Can you work these out from the model? Positions are in its coordinate system, mm. Give positions to 0.01 mm unless a question says otherwise; leave off trailing zeros. Loops run counter-clockwise (first coordinate to the right, second up) from the corner with the lowest first, then second, coordinate; pieces in that order, holes last. Notation, with made-up numbers: (24.25, -34.5) - (31.25, -34.5) arc R32 ccw to (31.25, -3.5) - close; hole circle Ø1 at (2, 52). An arc over 180 degrees is marked (long way). Use a Markdown table: item, result. Add a question column.
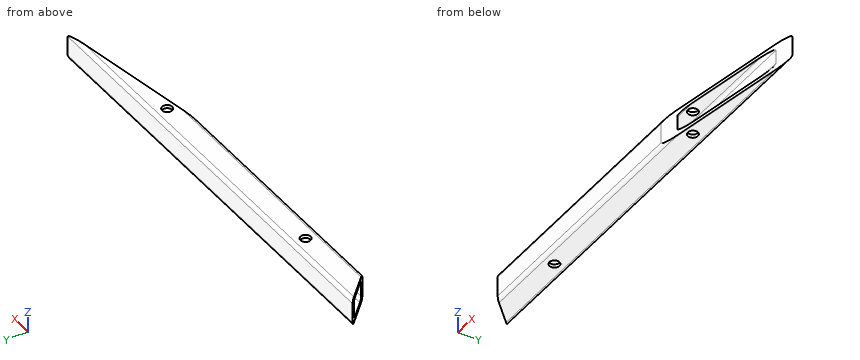
```python
from build123d import *

# Parameters (mm, degrees)
BOSS_EXTRUDE1_DEPTH = 418.338
SKETCH2_R           = 4.7625
CUT_EXTRUDE1_DEPTH  = 420.87736572


with BuildPart() as part:
    # Sketch1 → Boss-Extrude1 (new body)
    with BuildSketch(Plane(origin=(0, 0, 0), x_dir=(0, 0, -1), z_dir=(1, 0, 0))):
        with BuildLine():
            Line((3.302, 0), (22.098, 0))
            ThreePointArc((22.098, 0), (24.432866591, 0.967133409), (25.4, 3.302))
            Line((25.4, 3.302), (25.4, 22.098))
            ThreePointArc((25.4, 22.098), (24.432866591, 24.432866591), (22.098, 25.4))
            Line((22.098, 25.4), (3.302, 25.4))
            ThreePointArc((3.302, 25.4), (0.967133409, 24.432866591), (0, 22.098))
            Line((0, 22.098), (0, 3.302))
            ThreePointArc((0, 3.302), (0.967133409, 0.967133409), (3.302, 0))
        make_face()
        with BuildLine():
            Line((6.223, 3.175), (19.177, 3.175))
            ThreePointArc((19.177, 3.175), (21.332261469, 4.067738531), (22.225, 6.223))
            Line((22.225, 6.223), (22.225, 19.177))
            ThreePointArc((22.225, 19.177), (21.332261469, 21.332261469), (19.177, 22.225))
            Line((19.177, 22.225), (6.223, 22.225))
            ThreePointArc((6.223, 22.225), (4.067738531, 21.332261469), (3.175, 19.177))
            Line((3.175, 19.177), (3.175, 6.223))
            ThreePointArc((3.175, 6.223), (4.067738531, 4.067738531), (6.223, 3.175))
        make_face(mode=Mode.SUBTRACT)
    extrude(amount=BOSS_EXTRUDE1_DEPTH)

    # Sketch2 → Cut-Extrude1 (cut, through all)
    with BuildSketch(Plane.XY):
        with Locations((88.9, 12.7)):
            Circle(SKETCH2_R)
        with Locations((292.1, 12.7)):
            Circle(SKETCH2_R)
        Polygon((0, 0), (0, 25.4), (25.4, 0), align=None)
        Polygon((418.338, 0), (265.303, 0), (418.338, 25.4), align=None)
    extrude(amount=-CUT_EXTRUDE1_DEPTH, mode=Mode.SUBTRACT)


solid = part.part
```
1. Suppose I cut it at B-B (x = 88.9). List the corners of the cut face in (y, z) for me (1 decimal), and give its area (3 significant figures).
2. Please list where these lines run through material, in increasing order: line 1 along Z through (x, y) = (230, 13.5) (3 decimals); line 2 along Y through (x, z) = (88.9, -23.3); line 3 along Y through (x, z) = (292.1, -0.85). Write a range as [from, to].
3. Will these pins go through, and if not, where does the flat tip stop? P1, Ø5, axis at x = 321, z = -7.5, coming from the -Y side; P2, Ø6, axis at x = 352.5, y = 14, coming from the -Z side.
4. Suppose I cut it at A-A (z = -10.25). List the corners of the cut face in (x, y) for me (3 decimals).
5. Suppose I cut it at D-D (x = 292.1). List the corners of the cut face in (y, z) for me (1 decimal), and give its area (3 significant figures).
6. Suppose I cut it at C-C (x = 189). List the corners of the cut face in (y, z) for me (3 decimals), and give its area (3 significant figures).
Results below:
| question | item | result |
|---|---|---|
| 1 | outline | (0, -22.1) arc R3.3 ccw to (3.3, -25.4) - (7.9, -25.4) - (7.9, -22.2) - (6.2, -22.2) arc R3 cw to (3.2, -19.2) - (3.2, -6.2) arc R3 cw to (6.2, -3.2) - (7.9, -3.2) - (7.9, 0) - (3.3, 0) arc R3.3 ccw to (0, -3.3) - close; (17.5, -25.4) - (22.1, -25.4) arc R3.3 ccw to (25.4, -22.1) - (25.4, -3.3) arc R3.3 ccw to (22.1, 0) - (17.5, 0) - (17.5, -3.2) - (19.2, -3.2) arc R3 cw to (22.2, -6.2) - (22.2, -19.2) arc R3 cw to (19.2, -22.2) - (17.5, -22.2) - close |
| 1 | area | 220 mm² |
| 2 | line 1 | [-25.4, -22.225], [-3.175, 0] |
| 2 | line 2 | [0.23, 7.94], [17.46, 25.17] |
| 2 | line 3 | [4.45, 7.94], [17.46, 24.31] |
| 3 | P1 | y = 21.97 |
| 3 | P2 | z = -25.4 |
| 4 | outline | (0, 25.4) - (3.175, 22.225) - (399.209, 22.225) - (418.338, 25.4) - close; (22.225, 3.175) - (25.4, 0) - (265.303, 0) - (284.432, 3.175) - close |
| 5 | outline | (4.4, -25.4) - (7.9, -25.4) - (7.9, -22.2) - (6.2, -22.2) arc R3 cw to (4.4, -21.7) - close; (4.4, -3.7) arc R3 cw to (6.2, -3.2) - (7.9, -3.2) - (7.9, 0) - (4.4, 0) - close; (17.5, -25.4) - (22.1, -25.4) arc R3.3 ccw to (25.4, -22.1) - (25.4, -3.3) arc R3.3 ccw to (22.1, 0) - (17.5, 0) - (17.5, -3.2) - (19.2, -3.2) arc R3 cw to (22.2, -6.2) - (22.2, -19.2) arc R3 cw to (19.2, -22.2) - (17.5, -22.2) - close |
| 5 | area | 133 mm² |
| 6 | outline | (0, -22.098) arc R3.302 ccw to (3.302, -25.4) - (22.098, -25.4) arc R3.302 ccw to (25.4, -22.098) - (25.4, -3.302) arc R3.302 ccw to (22.098, 0) - (3.302, 0) arc R3.302 ccw to (0, -3.302) - close; hole (3.175, -19.177) arc R3.048 ccw to (6.223, -22.225) - (19.177, -22.225) arc R3.048 ccw to (22.225, -19.177) - (22.225, -6.223) arc R3.048 ccw to (19.177, -3.175) - (6.223, -3.175) arc R3.048 ccw to (3.175, -6.223) - close |
| 6 | area | 281 mm² |
